Geometry: final body of the model. Coordinates: model frame, mm. Face numbers are marked on the shaded views. A direction names the side the tool comes from. Round coordinates to 2 decimals unless told otherwise and drop trailing zeros. Order: outer loops, then holes, each group sorted by start corner. A loop starts at its lowest first (then second) coordinate and runs counter-clockwise, first axis right, second up. Notation, with made-up numbers: M -21,-9 L -15,-9 A15 cw -15,-4 Z; hole C 36.25,68.25 d8. An arc over 180 degrees is marked long. Put each result on its own line as item: value. Start each with the question number.
1) Draft query along Z for the marked faces 1 and 2. Return one class per face: pulls with the +Z half, pulls with the -Z half, needs draft (parallel to the pull), parting line crosses it, or undercut.
2) Access query for the marked faces 3, 4 and 5. Directions: +Z, -Z, +X, -X, +Y, -Y. A direction counts if a zero-diameter tool reaches every point of the face in a straight line with its end or side. Return the directions, or none.
3) Section B-B, the plane x = 0. Return loops of the section in (y, z).
4) Material intervals for probe 1 along Z at (x, y) = (0, 10.5); probe 2 along X at (y, z) = (-11, -422); probe 3 along Z at (x, y) = (168.5, -6), sorted ascending. Write a range as [from, to].
5) Section A-A, the plane z = 0. Return loops of the section in (x, y).
6) First-contact query: P1, Ø5, axis at x = 254.5, y = 9.5, coming from the +Z side; P2, Ø10, axis at y = 8.5, z = 398, coming from the -X side; P3, Ø8, axis at y = -6, z = -171, coming from the +X side. Flat tips, straight axial feed; report the tip coordinate or a pass-through.
7) Section D-D, the plane x = 236.5. Return loops of the section in (y, z), then the cut area to 3 significant figures.
8) Section C-C, the plane y = -13. Count the separate pieces of the cut face and the enclosed holes in it, then the cut area to 3 significant figures.
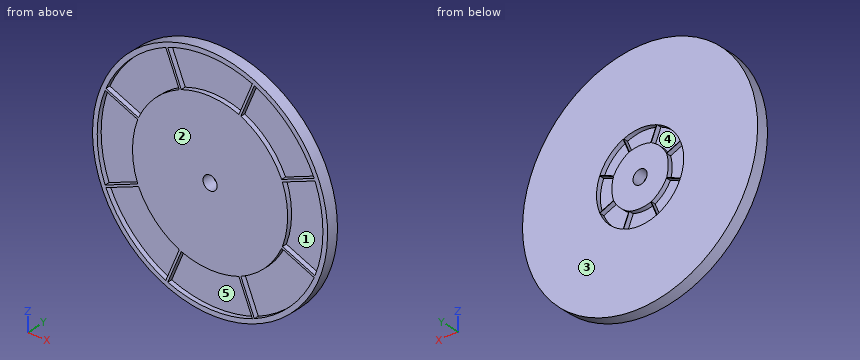
from build123d import *

# Parameters (mm, degrees)
SKETCH1_W          = 470
SKETCH1_H          = 50
CUT_EXTRUDE1_DEPTH = 20
CUT_EXTRUDE2_DEPTH = 20


with BuildPart() as part:
    # Sketch1 → Revolve1 (revolve)
    with BuildSketch(Plane(origin=(0, 0, 0), x_dir=(0, 0, -1), z_dir=(1, 0, 0))):
        with Locations((-265, 0)):
            Rectangle(SKETCH1_W, SKETCH1_H)
    revolve(axis=Axis((0, 285.555555556, 0), (0, -1, 0)))

    # Sketch2 → Cut-Extrude1 (cut)
    with BuildSketch(Plane.XZ.offset(25)):
        with BuildLine():
            Line((-180, 446.476151588), (-122.573000413, 307.835110337))
            ThreePointArc((-122.573000413, 307.835110337), (0, 330), (122.573000413, 307.835110337))
            Line((122.573000413, 307.835110337), (180, 446.476151588))
            ThreePointArc((180, 446.476151588), (0, 480), (-180, 446.476151588))
        make_face()
        with BuildLine():
            Line((188.427093812, 442.985535039), (131.000094225, 304.344493789))
            ThreePointArc((131.000094225, 304.344493789), (233.345237792, 233.345237792), (304.344493789, 131.000094225))
            Line((304.344493789, 131.000094225), (442.985535039, 188.427093812))
            ThreePointArc((442.985535039, 188.427093812), (339.41125497, 339.41125497), (188.427093812, 442.985535039))
        make_face()
        with BuildLine():
            Line((446.476151588, 180), (307.835110337, 122.573000413))
            ThreePointArc((307.835110337, 122.573000413), (330, 0), (307.835110337, -122.573000413))
            Line((307.835110337, -122.573000413), (446.476151588, -180))
            ThreePointArc((446.476151588, -180), (480, 0), (446.476151588, 180))
        make_face()
        with BuildLine():
            Line((442.985535039, -188.427093812), (304.344493789, -131.000094225))
            ThreePointArc((304.344493789, -131.000094225), (233.345237792, -233.345237792), (131.000094225, -304.344493789))
            Line((131.000094225, -304.344493789), (188.427093812, -442.985535039))
            ThreePointArc((188.427093812, -442.985535039), (339.41125497, -339.41125497), (442.985535039, -188.427093812))
        make_face()
        with BuildLine():
            Line((180, -446.476151588), (122.573000413, -307.835110337))
            ThreePointArc((122.573000413, -307.835110337), (0, -330), (-122.573000413, -307.835110337))
            Line((-122.573000413, -307.835110337), (-180, -446.476151588))
            ThreePointArc((-180, -446.476151588), (0, -480), (180, -446.476151588))
        make_face()
        with BuildLine():
            Line((-188.427093812, -442.985535039), (-131.000094225, -304.344493789))
            ThreePointArc((-131.000094225, -304.344493789), (-233.345237792, -233.345237792), (-304.344493789, -131.000094225))
            Line((-304.344493789, -131.000094225), (-442.985535039, -188.427093812))
            ThreePointArc((-442.985535039, -188.427093812), (-339.41125497, -339.41125497), (-188.427093812, -442.985535039))
        make_face()
        with BuildLine():
            Line((-446.476151588, -180), (-307.835110337, -122.573000413))
            ThreePointArc((-307.835110337, -122.573000413), (-330, 0), (-307.835110337, 122.573000413))
            Line((-307.835110337, 122.573000413), (-446.476151588, 180))
            ThreePointArc((-446.476151588, 180), (-480, 0), (-446.476151588, -180))
        make_face()
        with BuildLine():
            Line((-442.985535039, 188.427093812), (-304.344493789, 131.000094225))
            ThreePointArc((-304.344493789, 131.000094225), (-233.345237792, 233.345237792), (-131.000094225, 304.344493789))
            Line((-131.000094225, 304.344493789), (-188.427093812, 442.985535039))
            ThreePointArc((-188.427093812, 442.985535039), (-339.41125497, 339.41125497), (-442.985535039, 188.427093812))
        make_face()
    extrude(amount=-CUT_EXTRUDE1_DEPTH, mode=Mode.SUBTRACT)

    # Sketch3 → Cut-Extrude2 (cut)
    with BuildSketch(Plane(origin=(0, 25, 0), x_dir=(1, 0, 0), z_dir=(0, 1, 0))):
        with BuildLine():
            Line((-45.632403393, 112.890460705), (-70, 171.719042916))
            ThreePointArc((-70, 171.719042916), (0, 185.438479556), (70, 171.719042916))
            Line((70, 171.719042916), (45.632403393, 112.890460705))
            ThreePointArc((45.632403393, 112.890460705), (0, 120), (-45.632403393, 112.890460705))
        make_face()
        with BuildLine():
            Line((112.092592177, 47.558628415), (170.921174388, 71.926225022))
            ThreePointArc((170.921174388, 71.926225022), (131.124806387, 131.124806387), (71.926225022, 170.921174388))
            Line((71.926225022, 170.921174388), (47.558628415, 112.092592177))
            ThreePointArc((47.558628415, 112.092592177), (84.852813742, 84.852813742), (112.092592177, 47.558628415))
        make_face()
        with BuildLine():
            Line((112.890460705, -45.632403393), (171.719042916, -70))
            ThreePointArc((171.719042916, -70), (185.438479556, 0), (171.719042916, 70))
            Line((171.719042916, 70), (112.890460705, 45.632403393))
            ThreePointArc((112.890460705, 45.632403393), (120, 0), (112.890460705, -45.632403393))
        make_face()
        with BuildLine():
            Line((47.558628415, -112.092592177), (71.926225022, -170.921174388))
            ThreePointArc((71.926225022, -170.921174388), (131.124806387, -131.124806387), (170.921174388, -71.926225022))
            Line((170.921174388, -71.926225022), (112.092592177, -47.558628415))
            ThreePointArc((112.092592177, -47.558628415), (84.852813742, -84.852813742), (47.558628415, -112.092592177))
        make_face()
        with BuildLine():
            Line((-45.632403393, -112.890460705), (-70, -171.719042916))
            ThreePointArc((-70, -171.719042916), (0, -185.438479556), (70, -171.719042916))
            Line((70, -171.719042916), (45.632403393, -112.890460705))
            ThreePointArc((45.632403393, -112.890460705), (0, -120), (-45.632403393, -112.890460705))
        make_face()
        with BuildLine():
            Line((-112.092592177, -47.558628415), (-170.921174388, -71.926225022))
            ThreePointArc((-170.921174388, -71.926225022), (-131.124806387, -131.124806387), (-71.926225022, -170.921174388))
            Line((-71.926225022, -170.921174388), (-47.558628415, -112.092592177))
            ThreePointArc((-47.558628415, -112.092592177), (-84.852813742, -84.852813742), (-112.092592177, -47.558628415))
        make_face()
        with BuildLine():
            Line((-112.890460705, 45.632403393), (-171.719042916, 70))
            ThreePointArc((-171.719042916, 70), (-185.438479556, 0), (-171.719042916, -70))
            Line((-171.719042916, -70), (-112.890460705, -45.632403393))
            ThreePointArc((-112.890460705, -45.632403393), (-120, 0), (-112.890460705, 45.632403393))
        make_face()
        with BuildLine():
            Line((-47.558628415, 112.092592177), (-71.926225022, 170.921174388))
            ThreePointArc((-71.926225022, 170.921174388), (-131.124806387, 131.124806387), (-170.921174388, 71.926225022))
            Line((-170.921174388, 71.926225022), (-112.092592177, 47.558628415))
            ThreePointArc((-112.092592177, 47.558628415), (-84.852813742, 84.852813742), (-47.558628415, 112.092592177))
        make_face()
    extrude(amount=-CUT_EXTRUDE2_DEPTH, mode=Mode.SUBTRACT)


solid = part.part
Result sheet:
1. face 1: undercut
1. face 2: needs draft
2. face 3: +Z, -Z, +X, -X, +Y
2. face 4: +Y
2. face 5: -Y
3. outline: M -25,-500 L 25,-500 L 25,-185.44 L 5,-185.44 L 5,-120 L 25,-120 L 25,-30 L -25,-30 L -25,-330 L -5,-330 L -5,-480 L -25,-480 Z; M -25,30 L 25,30 L 25,120 L 5,120 L 5,185.44 L 25,185.44 L 25,500 L -25,500 L -25,480 L -5,480 L -5,330 L -25,330 Z
4. probe 1: z = [-500, -185.44], [-120, -30], [30, 120], [185.44, 500]
4. probe 2: x = [-268.17, -230.36], [-179.73, -169.86], [169.86, 179.73], [230.36, 268.17]
4. probe 3: z = [-470.75, -450.75], [-418.71, -394.88], [-284.42, 284.42], [394.88, 418.71], [450.75, 470.75]
5. outline: M -500,-25 L -480,-25 L -480,-5 L -330,-5 L -330,-25 L -30,-25 L -30,25 L -120,25 L -120,5 L -185.44,5 L -185.44,25 L -500,25 Z; M 30,-25 L 330,-25 L 330,-5 L 480,-5 L 480,-25 L 500,-25 L 500,25 L 185.44,25 L 185.44,5 L 120,5 L 120,25 L 30,25 Z
6. P1: stops at z = 431.85
6. P2: stops at x = -309.11
6. P3: stops at x = 471.29
7. outline: M -25,-440.53 L 25,-440.53 L 25,440.53 L -25,440.53 L -25,418.5 L -5,418.5 L -5,230.15 L -25,230.15 L -25,-230.15 L -5,-230.15 L -5,-418.5 L -25,-418.5 Z
7. area: 36,500 mm2
8. separate pieces: 1
8. enclosed holes: 9
8. area: 411,000 mm2
